Build history of the part. All positions in model axes, mm. Face numbers are marked on the shaded views. Give positions to 0.01 mm unless a question says otherwise; leave off trailing zeros. Loops run counter-clockwise (first coordinate to the right, second up) from the corner with the lowest first, then second, coordinate; pieces in that order, holes last. Notation, with made-up numbers: (33.25, 84) -> (65.25, 84) arc R27 ccw to (65.25, 121) -> close; hole circle Ø10 at (-27, 39). An arc over 180 degrees is marked (long way). Answer in a Markdown table with one row per item. Add a question column.
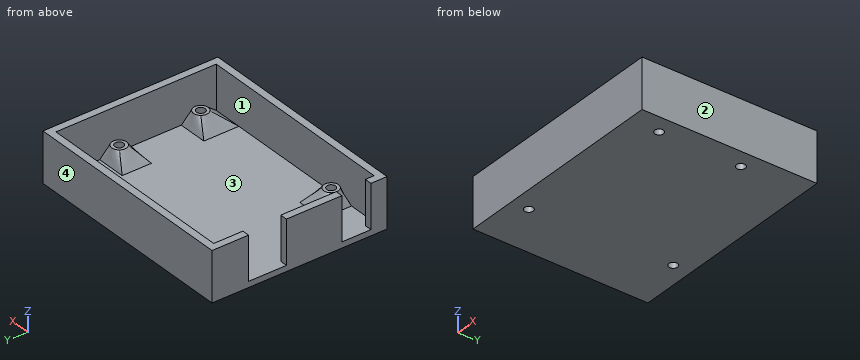
from build123d import *

# Parameters (mm, degrees)
F0_W      = 75
F0_H      = 60
F1_DEPTH  = 2
F2_W      = 75
F2_H      = 60
F2_W_2    = 70
F2_H_2    = 55
F3_DEPTH  = 15
F4_W      = 10
F4_H      = 10
F4_H_2    = 12
F11_D     = 3
F12_W     = 10
F12_H     = 15
F12_W_2   = 13
F13_DEPTH = 2.5


with BuildPart() as f1:
    # F0 (on Top) → F1 (new body)
    with BuildSketch(Plane.XY):
        Rectangle(F0_W, F0_H)
    extrude(amount=F1_DEPTH)

    # F2 (on face) → F3 (join)
    with BuildSketch(Plane.XY.offset(2)):
        Rectangle(F2_W, F2_H)
        Rectangle(F2_W_2, F2_H_2, mode=Mode.SUBTRACT)
    extrude(amount=F3_DEPTH)

    # F4 (on face) → F7 section 0
    with BuildSketch(Plane.XY.offset(2)):
        with Locations((-20, 22.5)):
            Rectangle(F4_W, F4_H)
    # F6 (on offset) → F7 section 1
    with BuildSketch(Plane.XY.offset(7)):
        with BuildLine():
            ThreePointArc((-20.293224, 22.258062), (-18.819991, 21.520563), (-17.207788, 21.859863))
            ThreePointArc((-17.207788, 21.859863), (-16.000779, 23.937586), (-17.102572, 26.072968))
            ThreePointArc((-17.102572, 26.072968), (-18.99862, 26.449771), (-20.596534, 25.361817))
            ThreePointArc((-20.596534, 25.361817), (-20.988147, 23.756849), (-20.293224, 22.258062))
        make_face()
    loft()

    # F4 (on face) → F8 section 0
    with BuildSketch(Plane.XY.offset(2)):
        with Locations((30, 7.5)):
            Rectangle(F4_W, F4_H)
    # F6 (on offset) → F8 section 1
    with BuildSketch(Plane.XY.offset(7)):
        with BuildLine():
            ThreePointArc((29.818347, 6.650123), (31.321839, 6.006356), (32.901582, 6.429838))
            ThreePointArc((32.901582, 6.429838), (33.991199, 8.290416), (33.227758, 10.306891))
            ThreePointArc((33.227758, 10.306891), (31.280438, 10.99034), (29.482742, 9.976709))
            ThreePointArc((29.482742, 9.976709), (29.012626, 8.249059), (29.818347, 6.650123))
        make_face()
    loft()

    # F4 (on face) → F9 section 0
    with BuildSketch(Plane.XY.offset(2)):
        with Locations((30, -21.5)):
            Rectangle(F4_W, F4_H_2)
    # F6 (on offset) → F9 section 1
    with BuildSketch(Plane.XY.offset(7)):
        with BuildLine():
            ThreePointArc((29.529474, -17.961486), (29.007923, -19.698875), (29.798415, -21.331559))
            ThreePointArc((29.798415, -21.331559), (31.356554, -21.995881), (32.980542, -21.514447))
            ThreePointArc((32.980542, -21.514447), (33.997404, -19.613892), (33.157749, -17.628672))
            ThreePointArc((33.157749, -17.628672), (31.271639, -17.010452), (29.529474, -17.961486))
        make_face()
    loft()

    # F4 (on face) → F10 section 0
    with BuildSketch(Plane.XY.offset(2)):
        with Locations((-20, -22.5)):
            Rectangle(F4_W, F4_H)
    # F6 (on offset) → F10 section 1
    with BuildSketch(Plane.XY.offset(7)):
        with BuildLine():
            ThreePointArc((-19.030994, -21.977126), (-20.71328, -21.509114), (-22.291516, -22.256305))
            ThreePointArc((-22.291516, -22.256305), (-22.998858, -23.92446), (-22.393571, -25.632296))
            ThreePointArc((-22.393571, -25.632296), (-20.449964, -26.499499), (-18.54262, -25.555205))
            ThreePointArc((-18.54262, -25.555205), (-18.022967, -23.661909), (-19.030994, -21.977126))
        make_face()
    loft()

    # F11 (through all)
    with Locations(Plane.XY.offset(7)):
        with Locations((-18.5, 24), (31.5, 8.5), (31.5, -19.5), (-20.5, -24)):
            Hole(F11_D / 2)

    # F12 (on face) → F13 (cut, through all)
    with BuildSketch(Plane.YZ.offset(-35)):
        with Locations((-19.5, 9.5)):
            Rectangle(F12_W, F12_H)
        with Locations((11, 9.5)):
            Rectangle(F12_W_2, F12_H)
    extrude(amount=-F13_DEPTH, mode=Mode.SUBTRACT)


solid = f1.part
(1) Two-plate mould, pull along Y, no slides. Class the marked faces 1, 2, 3 and 4: released by +Y, released by -Y, zero draft, split by the parting line, or undercut.
(2) Wall check: line 1 along Y through (x, z) = (31.5, 1.5); line 2 along Y through (x, z) = (-23.5, 11.5); line 3 along X through (y, z) = (-12.5, 13.5). Give the ranges that are in metal, low to high. Write a range as from..to.
(3) Flat gauge pins, fed straight in: pin 1 Ø1.5 at (x, y) = (-19.5, -23.5) entering from +Z; pin 2 Ø2.5 at (x, y) = (31.5, -19.5) entering from +Z; pin 3 Ø1.5 at (x, y) = (25, 3) entering from +Z; pin 4 Ø5 at (x, y) = (-19.5, 19) entering from +Z. Where does each tip first touch, or does it go through?
(4) Saw through at B-B, the plane y = 1.5. List the corners of the cut face in (x, z).
(5) Saw through at C-C, the plane x = 0. List the corners of the cut face in (y, z).
(6) Saw through at A-A, the plane z = 15.25. List the corners of the cut face in (x, y), then the cut area to 4 significant figures.
(7) Saw through at D-D, the plane x = 31.5. State how many separate pieces and enclosed holes the cut face has, then the cut area to 3 significant figures.
Worked answers:
| question | item | result |
|---|---|---|
| 1 | face 1 | undercut |
| 1 | face 2 | zero draft |
| 1 | face 3 | undercut |
| 1 | face 4 | released by +Y |
| 2 | line 1 | -30..-21, -18..7, 10..30 |
| 2 | line 2 | -30..-27.5, 27.5..30 |
| 2 | line 3 | -37.5..-35, 35..37.5 |
| 3 | pin 1 | z = 7 |
| 3 | pin 2 | through |
| 3 | pin 3 | z = 2.77 |
| 3 | pin 4 | z = 6.88 |
| 4 | outline | (-37.5, 0) -> (37.5, 0) -> (37.5, 17) -> (35, 17) -> (35, 2) -> (-35, 2) -> (-35, 17) -> (-37.5, 17) -> close |
| 5 | outline | (-30, 0) -> (30, 0) -> (30, 17) -> (27.5, 17) -> (27.5, 2) -> (-27.5, 2) -> (-27.5, 17) -> (-30, 17) -> close |
| 6 | outline | (-37.5, -30) -> (37.5, -30) -> (37.5, 30) -> (-37.5, 30) -> (-37.5, 17.5) -> (-35, 17.5) -> (-35, 27.5) -> (35, 27.5) -> (35, -27.5) -> (-35, -27.5) -> (-35, -24.5) -> (-37.5, -24.5) -> close; (-37.5, -14.5) -> (-35, -14.5) -> (-35, 4.5) -> (-37.5, 4.5) -> close |
| 6 | area | 592.5 mm^2 |
| 7 | separate pieces | 3 |
| 7 | enclosed holes | 0 |
| 7 | area | 233 mm^2 |
